Input: part model. Units: mm. Frame: model coordinates. Face numbers are marked on the shaded views. A direction names the side the tool comes from. Coordinates: 2 decimals unless noted, no trailing zeros. Write each loop counter-clockwise with the first axis right and the second up, starting at its lowest first coordinate (ties: lowest second). Pieces come first, ordered by that corner, then holes. Notation, with made-up numbers: (-25.5, 7) -> (-8.5, 7) arc R14 cw to (-8.5, 16) -> close; hole circle Ø9 at (23, 21). An arc over 180 degrees is marked (long way). Use one line per item in the form item = value. Start each with the question number.
(1) Set-up query: the marked faces 1, 2 and 3. Return all of +Z, -Z, +X, -X, +Y, -Y with unobstructed straight access to the full face (end or side cutting, diameter ignored); none if empty.
(2) Cut plane A-A on x = -3.5. Return the cut outline in (y, z), plus the area to 3 significant figures.
(3) Pull-direction query (X, two-part tool) for the marked faces 4, 5 and 6; classes: released by +X, released by -X, zero draft, split by the parting line, or undercut.
(4) Ray query, line 1 along Z through (x, y) = (-0.25, 3.5); line 2 along Z through (x, y) = (-0.25, -3.75); line 3 along Y through (x, z) = (0, 5.8). Return the intervals inside material, ascending.
(5) First-contact query: pin 1 (5 mm diameter, centred on x = 0, y = 0, fed in from +Z); pin 2 (2.5 mm diameter, centred on x = 0, y = 0, fed in from +Z); pin 3 (1.2 mm diameter, centred on x = -0.03, z = -3.99, fed in from -Y); pin 4 (6 mm diameter, centred on x = 4, z = 6, fed in from +Y). Flat tips, straight axial feed; report the tip coordinate or a pass-through.
```python
from build123d import *

# Parameters (mm, degrees)
SKETCH1_R           = 1.7653
BOSS_EXTRUDE1_DEPTH = 9.398
SKETCH2_R           = 5.334
SKETCH2_R_2         = 1.5875
BOSS_EXTRUDE2_DEPTH = 1.27
BOSS_EXTRUDE3_START = -1.27
SKETCH3_R           = 5.334
SKETCH3_R_2         = 1.5875
BOSS_EXTRUDE3_DEPTH = 1.27
SKETCH4_R           = 5.302265601
BOSS_EXTRUDE4_DEPTH = 5.08
SKETCH5_R           = 1.016
CUT_EXTRUDE1_DEPTH  = 7.62
SKETCH7_R           = 1.5875
CUT_EXTRUDE3_DEPTH  = 18.461460878


with BuildPart() as part:
    # Sketch1 → Boss-Extrude1 (new body)
    with BuildSketch(Plane.XY.offset(7.9502)):
        with BuildLine():
            Line((-2.508852776, -0.3048), (-2.933400151, -0.549912542))
            ThreePointArc((-2.933400151, -0.549912542), (-2.838428173, -0.92226122), (-2.696401056, -1.279320756))
            Line((-2.696401056, -1.279320756), (-2.208861477, -1.228078282))
            ThreePointArc((-2.208861477, -1.228078282), (-2.04462865, -1.485509668), (-1.850547587, -1.721255042))
            Line((-1.850547587, -1.721255042), (-2.049940092, -2.169097939))
            ThreePointArc((-2.049940092, -2.169097939), (-1.754245085, -2.41451122), (-1.429468404, -2.619897008))
            Line((-1.429468404, -2.619897008), (-1.06516017, -2.291872401))
            ThreePointArc((-1.06516017, -2.291872401), (-0.78097865, -2.403605134), (-0.485396118, -2.480249161))
            Line((-0.485396118, -2.480249161), (-0.383472592, -2.959761649))
            ThreePointArc((-0.383472592, -2.959761649), (0, -2.9845), (0.383472592, -2.959761649))
            Line((0.383472592, -2.959761649), (0.485396118, -2.480249161))
            ThreePointArc((0.485396118, -2.480249161), (0.78097865, -2.403605134), (1.06516017, -2.291872401))
            Line((1.06516017, -2.291872401), (1.429468404, -2.619897008))
            ThreePointArc((1.429468404, -2.619897008), (1.754245085, -2.41451122), (2.049940092, -2.169097939))
            Line((2.049940092, -2.169097939), (1.850547587, -1.721255042))
            ThreePointArc((1.850547587, -1.721255042), (2.04462865, -1.485509668), (2.208861477, -1.228078282))
            Line((2.208861477, -1.228078282), (2.696401056, -1.279320756))
            ThreePointArc((2.696401056, -1.279320756), (2.838428173, -0.92226122), (2.933400151, -0.549912542))
            Line((2.933400151, -0.549912542), (2.508852776, -0.3048))
            ThreePointArc((2.508852776, -0.3048), (2.5273, 0), (2.508852776, 0.3048))
            Line((2.508852776, 0.3048), (2.933400151, 0.549912542))
            ThreePointArc((2.933400151, 0.549912542), (2.838428173, 0.92226122), (2.696401056, 1.279320756))
            Line((2.696401056, 1.279320756), (2.208861477, 1.228078282))
            ThreePointArc((2.208861477, 1.228078282), (2.04462865, 1.485509668), (1.850547587, 1.721255042))
            Line((1.850547587, 1.721255042), (2.049940092, 2.169097939))
            ThreePointArc((2.049940092, 2.169097939), (1.754245085, 2.41451122), (1.429468404, 2.619897008))
            Line((1.429468404, 2.619897008), (1.06516017, 2.291872401))
            ThreePointArc((1.06516017, 2.291872401), (0.78097865, 2.403605134), (0.485396118, 2.480249161))
            Line((0.485396118, 2.480249161), (0.383472592, 2.959761649))
            ThreePointArc((0.383472592, 2.959761649), (0, 2.9845), (-0.383472592, 2.959761649))
            Line((-0.383472592, 2.959761649), (-0.485396118, 2.480249161))
            ThreePointArc((-0.485396118, 2.480249161), (-0.78097865, 2.403605134), (-1.06516017, 2.291872401))
            Line((-1.06516017, 2.291872401), (-1.429468404, 2.619897008))
            ThreePointArc((-1.429468404, 2.619897008), (-1.754245085, 2.41451122), (-2.049940092, 2.169097939))
            Line((-2.049940092, 2.169097939), (-1.850547587, 1.721255042))
            ThreePointArc((-1.850547587, 1.721255042), (-2.04462865, 1.485509668), (-2.208861477, 1.228078282))
            Line((-2.208861477, 1.228078282), (-2.696401056, 1.279320756))
            ThreePointArc((-2.696401056, 1.279320756), (-2.838428173, 0.92226122), (-2.933400151, 0.549912542))
            Line((-2.933400151, 0.549912542), (-2.508852776, 0.3048))
            ThreePointArc((-2.508852776, 0.3048), (-2.5273, 0), (-2.508852776, -0.3048))
        make_face()
        with Locations(Location((0, 0, 0), (0, 0, 180))):
            Circle(SKETCH1_R, mode=Mode.SUBTRACT)
    extrude(amount=-BOSS_EXTRUDE1_DEPTH)

    # Sketch2 → Boss-Extrude2 (add)
    with BuildSketch(Plane.XY.offset(7.9502)):
        Circle(SKETCH2_R)
        Circle(SKETCH2_R_2, mode=Mode.SUBTRACT)
    extrude(amount=BOSS_EXTRUDE2_DEPTH)

    # Sketch3 → Boss-Extrude3 (add)
    with BuildSketch(Plane.XY.offset(3.8862).offset(BOSS_EXTRUDE3_START)):
        Circle(SKETCH3_R)
        Circle(SKETCH3_R_2, mode=Mode.SUBTRACT)
    extrude(amount=BOSS_EXTRUDE3_DEPTH)

    # Sketch4 → Boss-Extrude4 (add)
    with BuildSketch(Plane(origin=(0, 0, -1.4478), x_dir=(-1, 0, 0), z_dir=(0, 0, -1))):
        Circle(SKETCH4_R)
    extrude(amount=BOSS_EXTRUDE4_DEPTH)

    # Sketch5 → Cut-Extrude1 (cut)
    with BuildSketch(Plane(origin=(0, 0, 0), x_dir=(1, 0, 0), z_dir=(0, 1, 0))):
        with Locations(Location((-0.031734399, 3.9878, 0), (0, 0, 270))):
            Circle(SKETCH5_R)
    extrude(amount=-CUT_EXTRUDE1_DEPTH, mode=Mode.SUBTRACT)

    # Sketch7 → Cut-Extrude3 (cut, through all)
    with BuildSketch(Plane(origin=(0, 0, -6.5278), x_dir=(-1, 0, 0), z_dir=(0, 0, -1))):
        with Locations(Location((0, 0, 0), (0, 0, 180))):
            Circle(SKETCH7_R)
    extrude(amount=-CUT_EXTRUDE3_DEPTH, mode=Mode.SUBTRACT)


solid = part.part
```
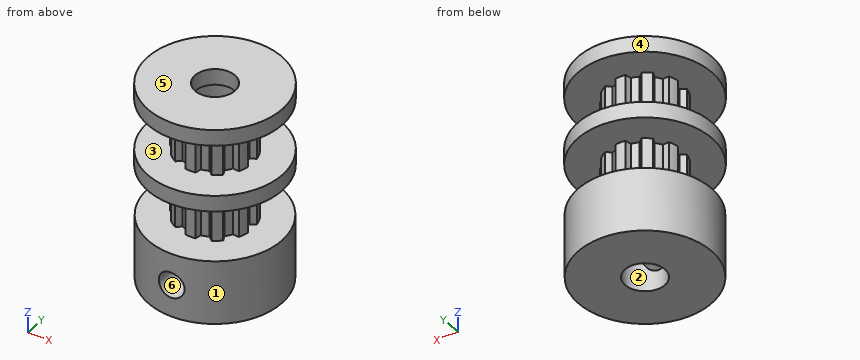
Values:
q1.face_1 = -Z
q1.face_2 = +Z, -Z
q1.face_3 = none
q2.outline = (-4.03, 2.62) -> (4.03, 2.62) -> (4.03, 3.89) -> (-4.03, 3.89) -> close; (-4.03, 7.95) -> (4.03, 7.95) -> (4.03, 9.22) -> (-4.03, 9.22) -> close; (-3.98, -6.53) -> (3.98, -6.53) -> (3.98, -1.45) -> (-3.98, -1.45) -> close
q2.area = 60.9 mm2
q3.face_4 = split by the parting line
q3.face_5 = zero draft
q3.face_6 = undercut
q4.line_1 = -6.53 to -1.45, 2.62 to 3.89, 7.95 to 9.22
q4.line_2 = -6.53 to -4.98, -3 to -1.45, 2.62 to 3.89, 7.95 to 9.22
q4.line_3 = -2.98 to -1.77, 1.77 to 2.98
q5.pin_1 = 9.22
q5.pin_2 = through
q5.pin_3 = 1.46
q5.pin_4 = 5.05
